Here's how the part is built. I have some questions about the finished solid (model axes, mm). A direction names the side the tool comes from. Give positions to 0.01 mm unless a question says otherwise; leave off trailing zeros. Loops run counter-clockwise (first coordinate to the right, second up) from the corner with the lowest first, then second, coordinate; pieces in that order, holes last. Notation, with made-up numbers: M 23.5,75 L 69.5,75 A19 ccw 69.5,101 Z; hole C 34.25,-27 d11. An arc over 180 degrees is marked long. Answer as CSV lines item,"result". Start each with the question number.
Item 1: I want a section at B-B on y = 24. List the corners of the cut face in (x, z) for me.
Item 2: Will these pins go through, and if not, where does the flat tip stop? P1, Ø1, axis at y = 28, z = -40.5, coming from the +X side; P2, Ø1, axis at y = -16.5, z = 24, coming from the +X side.
Item 3: I want a section at A-A on x = 17.5. List the corners of the cut face in (y, z) for me, plus the area to 3 significant figures.
Item 4: If we mould it in two halves opening along Z, with no side actions, what happens to faces 1 (the flat face through (4.762, -1, 0)), 2 (the cylindrical face through (1.106, 1.371, -40.642)), 3 (the flat face through (3, -97.955, 3))? For each: released by +Z, released by -Z, zero draft, split by the parting line, or undercut.
Item 5: I want a section at C-C on x = 46.5. List the corners of the cut face in (y, z) for me.
Item 6: If I drill on line 1 along Z through (x, y) = (14.5, -47); line 2 along Z through (x, y) = (49.5, 49); line 3 along X through (y, z) = (57, 32.5), over which ranges is the centre line in solid material (lowest first)? Write a range as from..to.
Item 7: For faces 4 (the flat face through (20, -1, -41.692)), 5 (the flat face through (29, -1, 37.644)), which set-ups out of +Z, -Z, +X, -X, +Y, -Y let a thin tool reach every point of the face, with its end or its side?
Item 8: I want a section at D-D on z = -11. List the corners of the cut face in (x, y) for me.
from build123d import *

# Parameters (mm, degrees)
F0_W     = 195.9098130465
F0_H     = 83.3830982447
F1_DEPTH = 4.7625
F2_W     = 195.9098130465
F2_H     = 3.2381750643
F3_DEPTH = 34.8488
F4_R     = 3.6792614691
F5_DEPTH = 3.175
F6_W     = 195.9098130465
F6_H     = 4.0477178991
F7_DEPTH = 49.53
F8_R     = 5.08


with BuildPart() as f1:
    # F0 (on Right) → F1 (new body)
    with BuildSketch(Plane.YZ):
        Rectangle(F0_W, F0_H)
    extrude(amount=F1_DEPTH)

    # F2 (on face) → F3 (join)
    with BuildSketch(Plane.YZ.offset(4.7625)):
        with Locations((0, -40.0724615902)):
            Rectangle(F2_W, F2_H)
    extrude(amount=F3_DEPTH)

    # F4
    f4_edges = [f1.edges().sort_by_distance(p)[0] for p in [
        (0, 0, -41.691549),
    ]]
    fillet(f4_edges, radius=F4_R)

    # F5 (cut): a face of the model
    f5_faces = [f1.faces().sort_by_distance(p)[0] for p in [
        (39.6113, 0, -40.0724615902),
    ]]
    extrude(f5_faces, amount=-F5_DEPTH, mode=Mode.SUBTRACT)

    # F6 (on face) → F7 (join)
    with BuildSketch(Plane.YZ.offset(4.7625)):
        with Locations((0, 39.6676901728)):
            Rectangle(F6_W, F6_H)
    extrude(amount=F7_DEPTH)

    # F8
    f8_edges = [f1.edges().sort_by_distance(p)[0] for p in [
        (0, 0, 41.691549),
    ]]
    fillet(f8_edges, radius=F8_R)


solid = f1.part
Result:
1,outline,"M 0,-38.01 A3.68 ccw 3.68,-41.69 L 36.44,-41.69 L 36.44,-38.45 L 4.76,-38.45 L 4.76,37.64 L 54.29,37.64 L 54.29,41.69 L 5.08,41.69 A5.08 ccw 0,36.61 Z"
2,P1,"x = 36.44"
2,P2,"x = 4.76"
3,outline,"M -97.95,-41.69 L 97.95,-41.69 L 97.95,-38.45 L -97.95,-38.45 Z; M -97.95,37.64 L 97.95,37.64 L 97.95,41.69 L -97.95,41.69 Z"
3,area,"1,430 mm^2"
4,face 1,"undercut"
4,face 2,"released by -Z"
4,face 3,"zero draft"
5,outline,"M -97.95,37.64 L 97.95,37.64 L 97.95,41.69 L -97.95,41.69 Z"
6,line 1,"-41.69..-38.45, 37.64..41.69"
6,line 2,"37.64..41.69"
6,line 3,"0..4.76"
7,face 4,"-Z, +X, -X, +Y, -Y"
7,face 5,"+X, +Y, -Y"
8,outline,"M 0,-97.95 L 4.76,-97.95 L 4.76,97.95 L 0,97.95 Z"
